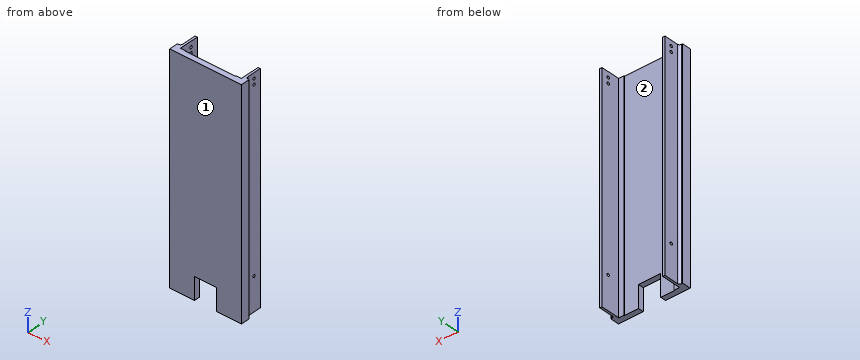
from build123d import *

# Parameters (mm, degrees)
BOSS_EXTRUDE1_DEPTH      = 400
SKETCH2_R                = 2.1
CUT_EXTRUDE3_DEPTH       = 10
SKETCH3_W                = 158.039132068
SKETCH3_H                = 497.98789011
CUT_EXTRUDE4_DEPTH       = 2
SKETCH4_W                = 4.8
SKETCH4_H                = 400
BOSS_EXTRUDE2_DEPTH      = 8
SKETCH5_R                = 1.2
CUT_EXTRUDE9_DEPTH       = 406.158043237
SKETCH9_R                = 1.225
CUT_EXTRUDE10_DEPTH      = 406.931077894
SKETCH10_W               = 4.8
SKETCH10_H               = 400
CUT_EXTRUDE11_DEPTH      = 5
BOSS_EXTRUDE3_START      = -15
SKETCH12_R               = 2.1
BOSS_EXTRUDE3_DEPTH      = 15
SKETCH13_W               = 6.18
SKETCH13_H               = 37.25
BOSS_EXTRUDE5_DEPTH      = 10
BOSS_EXTRUDE6_DEPTH      = 6.18
SKETCH15_R               = 1.05
CUT_EXTRUDE12_DEPTH      = 10
FILLET1_R                = 2
SKETCH16_W               = 4.8
SKETCH16_H               = 400
CUT_EXTRUDE13_DEPTH      = 2.5
CUT_EXTRUDE14_REACH      = 404.247
SKETCH17_R               = 1.16
CUT_EXTRUDE16_DEPTH      = 406.158043237
CUT_EXTRUDE16_DEPTH_BACK = 406.158043237
SKETCH18_R               = 1.225
CUT_EXTRUDE17_DEPTH      = 406.158043237
CUT_EXTRUDE17_DEPTH_BACK = 406.158043237
SKETCH20_R               = 1.225
SKETCH22_W               = 3
SKETCH22_H               = 15
CUT_EXTRUDE18_DEPTH      = 406.931077894
FILLET2_R                = 2
FILLET3_R                = 2
SKETCH24_W               = 20.2
SKETCH24_H               = 20
SKETCH24_W_2             = 2
SKETCH24_H_2             = 200
SKETCH24_W_3             = 3
CUT_EXTRUDE21_DEPTH      = 406.931077894


with BuildPart() as part:
    # Sketch1 → Boss-Extrude1 (new body)
    with BuildSketch(Plane.XY):
        Polygon((0, 0), (0, 25), (5, 25), (5, 5), (60.2, 5), (60.2, 25), (65.2, 25), (65.2, 0), align=None)
    extrude(amount=BOSS_EXTRUDE1_DEPTH)

    # Sketch2 → Cut-Extrude3 (cut)
    with BuildSketch(Plane(origin=(0, 5, 0), x_dir=(1, 0, 0), z_dir=(0, 1, 0))):
        with Locations(Location((32.6, -67.17, 0), (0, 0, 270))):
            Circle(SKETCH2_R)
        with Locations(Location((32.6, -96.92, 0), (0, 0, 270))):
            Circle(SKETCH2_R)
    extrude(amount=-CUT_EXTRUDE3_DEPTH, mode=Mode.SUBTRACT)

    # Sketch3 → Cut-Extrude4 (cut)
    with BuildSketch(Plane(origin=(0, 25, 0), x_dir=(1, 0, 0), z_dir=(0, 1, 0))):
        with Locations((44.123686713, -201.646240959)):
            Rectangle(SKETCH3_W, SKETCH3_H)
    extrude(amount=-CUT_EXTRUDE4_DEPTH, mode=Mode.SUBTRACT)

    # Sketch4 → Boss-Extrude2 (add)
    with BuildSketch(Plane(origin=(0, 5, 0), x_dir=(1, 0, 0), z_dir=(0, 1, 0))):
        with Locations((7.4, -200)):
            Rectangle(SKETCH4_W, SKETCH4_H)
        with Locations((57.8, -200)):
            Rectangle(SKETCH4_W, SKETCH4_H)
    extrude(amount=BOSS_EXTRUDE2_DEPTH)

    # Sketch5 → Cut-Extrude9 (cut, through all)
    with BuildSketch(Plane(origin=(5, 0, 0), x_dir=(0, 0, -1), z_dir=(1, 0, 0))):
        with Locations(Location((-395, 16.5, 0), (0, 0, 90))):
            Circle(SKETCH5_R)
        with Locations(Location((-390, 16.5, 0), (0, 0, 90))):
            Circle(SKETCH5_R)
        with Locations(Location((-10, 16.5, 0), (0, 0, 90))):
            Circle(SKETCH5_R)
        with Locations(Location((-5, 16.5, 0), (0, 0, 90))):
            Circle(SKETCH5_R)
    extrude(amount=-CUT_EXTRUDE9_DEPTH, mode=Mode.SUBTRACT)

    # Sketch9 → Cut-Extrude10 (cut, through all)
    with BuildSketch(Plane.ZY):
        with Locations((5, 16.5)):
            Circle(SKETCH9_R)
        with Locations((10, 16.5)):
            Circle(SKETCH9_R)
        with Locations((390, 16.5)):
            Circle(SKETCH9_R)
        with Locations((395, 16.5)):
            Circle(SKETCH9_R)
    extrude(amount=-CUT_EXTRUDE10_DEPTH, mode=Mode.SUBTRACT)

    # Sketch10 → Cut-Extrude11 (cut)
    with BuildSketch(Plane(origin=(0, 13, 0), x_dir=(1, 0, 0), z_dir=(0, 1, 0))):
        with Locations((7.4, -200)):
            Rectangle(SKETCH10_W, SKETCH10_H)
        with Locations((57.8, -200)):
            Rectangle(SKETCH10_W, SKETCH10_H)
    extrude(amount=-CUT_EXTRUDE11_DEPTH, mode=Mode.SUBTRACT)

    # Sketch12 → Boss-Extrude3 (add)
    with BuildSketch(Plane.XZ.offset(BOSS_EXTRUDE3_START)):
        with Locations(Location((32.6, 96.92, 0), (0, 0, 270))):
            Circle(SKETCH12_R)
        with Locations(Location((32.6, 67.17, 0), (0, 0, 270))):
            Circle(SKETCH12_R)
    extrude(amount=BOSS_EXTRUDE3_DEPTH)

    # Sketch13 → Boss-Extrude5 (add)
    with BuildSketch(Plane(origin=(0, 5, 0), x_dir=(1, 0, 0), z_dir=(0, 1, 0))):
        with Locations((32.6, -82.045)):
            Rectangle(SKETCH13_W, SKETCH13_H)
    extrude(amount=BOSS_EXTRUDE5_DEPTH)

    # Sketch14 → Boss-Extrude6 (add)
    with BuildSketch(Plane.ZY.offset(-29.51)):
        Polygon((70.92, 15), (75.32, 19.4), (88.77, 19.4), (93.17, 15), align=None)
    extrude(amount=-BOSS_EXTRUDE6_DEPTH)

    # Sketch15 → Cut-Extrude12 (cut)
    with BuildSketch(Plane.ZY.offset(-29.51)):
        with Locations((78.87, 16)):
            Circle(SKETCH15_R)
        with Locations((85.22, 16)):
            Circle(SKETCH15_R)
    extrude(amount=-CUT_EXTRUDE12_DEPTH, mode=Mode.SUBTRACT)

    # Fillet1
    fillet1_edges = [part.edges().sort_by_distance(p)[0] for p in [
        (29.51, 5, 82.045),
        (29.51, 10, 63.42),
        (32.6, 5, 100.67),
        (29.51, 10, 100.67),
        (35.69, 5, 82.045),
        (35.69, 10, 100.67),
        (32.6, 5, 63.42),
        (35.69, 10, 63.42),
    ]]
    fillet(fillet1_edges, radius=FILLET1_R)

    # Sketch16 → Cut-Extrude13 (cut)
    with BuildSketch(Plane(origin=(0, 8, 0), x_dir=(1, 0, 0), z_dir=(0, 1, 0))):
        with Locations((7.4, -200)):
            Rectangle(SKETCH16_W, SKETCH16_H)
        with Locations((57.8, -200)):
            Rectangle(SKETCH16_W, SKETCH16_H)
    extrude(amount=-CUT_EXTRUDE13_DEPTH, mode=Mode.SUBTRACT)

    # Sketch17 → Cut-Extrude14 (cut, up to next)
    with BuildSketch(Plane.ZY.offset(-29.51), mode=Mode.PRIVATE) as cut_extrude14_sk1:
        with Locations((78.87, 16)):
            Circle(SKETCH17_R)
    cut_extrude14_tool1 = extrude(cut_extrude14_sk1.sketch, amount=-CUT_EXTRUDE14_REACH, mode=Mode.PRIVATE) & part.part
    # Sketch17 → Cut-Extrude14 (cut, up to next)
    with BuildSketch(Plane.ZY.offset(-29.51), mode=Mode.PRIVATE) as cut_extrude14_sk2:
        with Locations((85.22, 16)):
            Circle(SKETCH17_R)
    cut_extrude14_tool2 = extrude(cut_extrude14_sk2.sketch, amount=-CUT_EXTRUDE14_REACH, mode=Mode.PRIVATE) & part.part
    add(cut_extrude14_tool1.solids().sort_by_distance((29.51, 16, 78.87))[0], mode=Mode.SUBTRACT)
    add(cut_extrude14_tool2.solids().sort_by_distance((29.51, 16, 85.22))[0], mode=Mode.SUBTRACT)

    # Sketch18 → Cut-Extrude16 (cut, two sides: drawn at the far end of the back side and taken through both)
    with BuildSketch(Plane.ZY.offset(-60.2).offset(-CUT_EXTRUDE16_DEPTH_BACK)):
        with Locations((170, 16.5)):
            Circle(SKETCH18_R)
    extrude(amount=CUT_EXTRUDE16_DEPTH + CUT_EXTRUDE16_DEPTH_BACK, mode=Mode.SUBTRACT)

    # Sketch20 → Cut-Extrude17 (cut, two sides: drawn at the far end of the back side and taken through both)
    with BuildSketch(Plane.ZY.offset(-60.2).offset(-CUT_EXTRUDE17_DEPTH_BACK)):
        with Locations((230, 16.5)):
            Circle(SKETCH20_R)
    extrude(amount=CUT_EXTRUDE17_DEPTH + CUT_EXTRUDE17_DEPTH_BACK, mode=Mode.SUBTRACT)

    # Sketch22 → Cut-Extrude18 (cut, through all)
    with BuildSketch(Plane(origin=(0, 0, 0), x_dir=(-1, 0, 0), z_dir=(0, 0, -1))):
        with Locations((-63.7, 15.5)):
            Rectangle(SKETCH22_W, SKETCH22_H)
        with Locations((-1.5, 15.5)):
            Rectangle(SKETCH22_W, SKETCH22_H)
    extrude(amount=-CUT_EXTRUDE18_DEPTH, mode=Mode.SUBTRACT)

    # Fillet2
    fillet2_edges = [part.edges().sort_by_distance(p)[0] for p in [
        (62.2, 8, 200),
    ]]
    fillet(fillet2_edges, radius=FILLET2_R)

    # Fillet3
    fillet3_edges = [part.edges().sort_by_distance(p)[0] for p in [
        (3, 8, 200),
    ]]
    fillet(fillet3_edges, radius=FILLET3_R)

    # Sketch24 → Cut-Extrude21 (cut, through all)
    with BuildSketch(Plane(origin=(0, 23, 0), x_dir=(1, 0, 0), z_dir=(0, 1, 0))):
        Polygon((0, 0), (0, -200), (22.5, -200), (42.7, -200), (60.2, -200), (60.2, 0), align=None)
        with Locations((32.6, -210)):
            Rectangle(SKETCH24_W, SKETCH24_H)
        with Locations((61.2, -100)):
            Rectangle(SKETCH24_W_2, SKETCH24_H_2)
        with Locations((63.7, -100)):
            Rectangle(SKETCH24_W_3, SKETCH24_H_2)
    extrude(amount=-CUT_EXTRUDE21_DEPTH, mode=Mode.SUBTRACT)


solid = part.part
The listing builds one solid part. Answer for the finished solid, in the listing's coordinates (mm). Face numbers are marked on the shaded views. Coordinates: 2 decimals unless noted, no trailing zeros. Write each loop counter-clockwise with the first axis right and the second up, starting at its lowest first coordinate (ties: lowest second). Pieces come first, ordered by that corner, then holes. Notation, with made-up numbers: M -35,22 L -11,22 A31 ccw -11,52 Z; hole C -31.5,6 d10. An arc over 180 degrees is marked long. Put each result on its own line as item: value. Start each with the question number.
1. Flat-ended cylindrical pins translate along their axes: P1, Ø0.8, axis at x = 0.5, z = 272.5, coming from the +Y side; P2, Ø3, axis at y = 16.5, z = 390, coming from the -X side; P3, Ø6, axis at x = 9.5, z = 326, coming from the +Y side. Find the tip coordinate at first contact, or state that the pin passes through.
2. A cutting plane is placed at A-A on z = 344.5. Write down the section's boundary in (x, y), then the cut area to 3 significant figures.
3. A cutting plane is placed at B-B on x = 33. Write down the section's boundary in (y, z).
4. Consider line 1 (X direction, y = 14.75, z = 294.5); line 2 (Y direction, x = 61.8, z = 230) (3 decimals); line 3 (X direction, y = 7.5, z = 222.5). Determine where each line is inside the solid, lowest interval first. Write a range as from..to.
5. For a pull along X with two mould halves and no side action, classify the marked faces 1 and 2 as pulls with the +X half, pulls with the -X half, needs draft (parallel to the pull), parting line crosses it, or undercut.
Resolved:
1. P1: stops at y = 8
1. P2: stops at x = 3
1. P3: stops at y = 5.5
2. outline: M 0,0 L 65.2,0 L 65.2,8 L 64.2,8 A2 cw 62.2,10 L 62.2,23 L 60.2,23 L 60.2,5.5 L 55.4,5.5 L 55.4,5 L 9.8,5 L 9.8,5.5 L 5,5.5 L 5,23 L 3,23 L 3,10 A2 cw 1,8 L 0,8 Z
2. area: 423 mm2
3. outline: M 0,220 L 5,220 L 5,400 L 0,400 Z
4. line 1: x = 3..5, 60.2..62.2
4. line 2: y = 0..15.275, 17.725..23
4. line 3: x = 0..5, 60.2..65.2
5. face 1: needs draft
5. face 2: undercut
